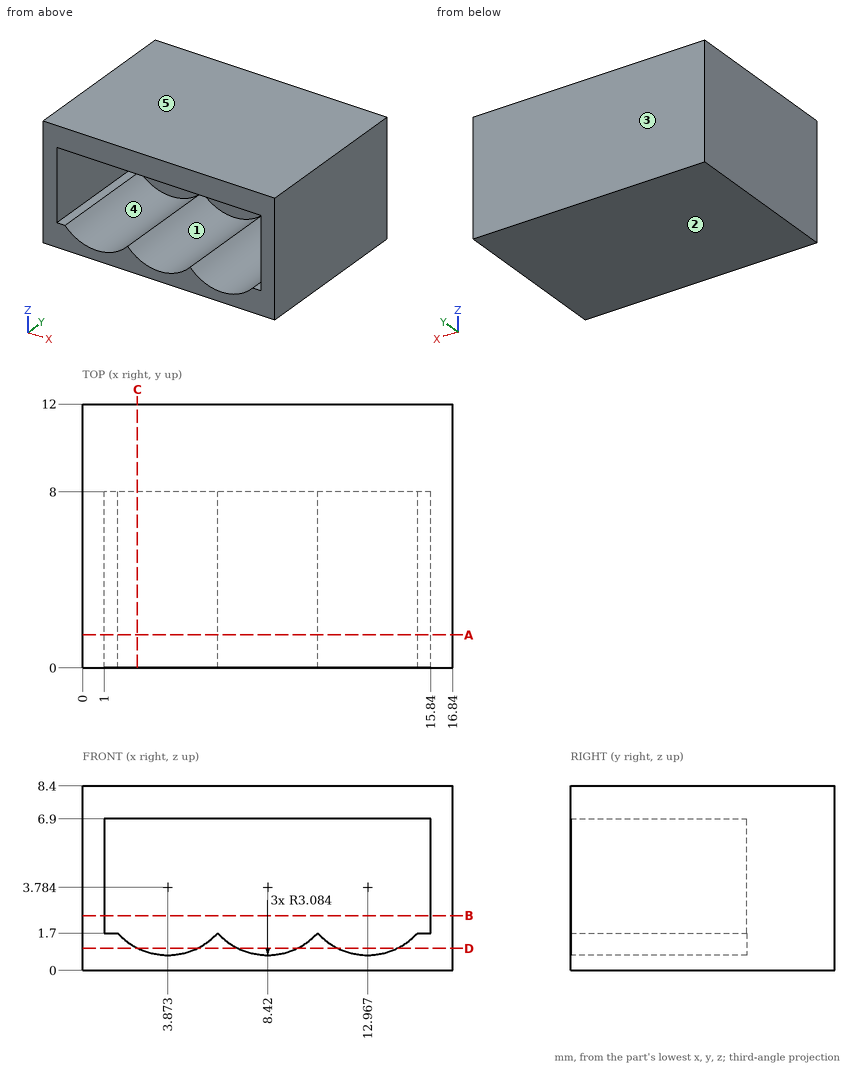
Job drawing, mm, ordinate dimensions from the low corner. One solid piece. A direction names the side the tool comes from. Give positions to 0.01 mm unless a question says otherwise; leave off trailing zeros. Write each loop counter-clockwise with the first axis right and the second up, starting at its lowest first coordinate (ties: lowest second). Pieces come first, ordered by that corner, then holes. Notation, with made-up numbers: M -35.75,-5.75 L -4.75,-5.75 A5 ccw -4.75,0.25 Z; hole C 58,-32 d5. An arc over 180 degrees is marked long. One line per item, written item: value. Start each with the question number.
Q1. Two-plate mould, pull along Z, no slides. Class the marked faces 3, 4 and 5: +Z half, -Z half, draft (parallel to the pull), parting line (faces both ways), or undercut.
Q2. Drop flat-ended pins along their axis: pin 1 Ø4 at (y, z) = (6, 4.5) entering from -X; pin 2 Ø1.9 at (x, z) = (6, 5) entering from -Y. Give the stop position or say it passes through.
Q3. Saw through at A-A, the plane y = 1.5. Write the cut outline in (x, z).
Q4. Saw through at B-B, the plane z = 2.5. Write the cut outline in (x, y).
Q5. Saw through at C-C, the plane x = 2.5. Write the cut outline in (y, z).
Q6. 3-axis set-ups, long thin cutter, end or side, ignore diameter. For the marked faces 1 and 2: which of +Z, -Z, +X, -X, +Y, -Y reach the whole face in a straight line?
Q7. Saw through at D-D, the plane z = 1. Write the cut outline in (x, y).
Q8. Probe probe 1 along X at (y, z) = (4.75, 5); probe 2 along Y at (x, z) = (9, 3.75); probe 3 along Z at (x, y) = (15, 7.25) (1 decimal). List the from-to ranges inside material, lowest first. Write a range as [from, to].
Output values:
1. face 3: draft
1. face 4: undercut
1. face 5: +Z half
2. pin 1: stops at x = 0
2. pin 2: stops at y = 8
3. outline: M 0,0 L 16.84,0 L 16.84,8.4 L 0,8.4 Z; hole M 1,1.7 L 1.6,1.7 A3.08 ccw 6.15,1.7 A3.08 ccw 10.69,1.7 A3.08 ccw 15.24,1.7 L 15.84,1.7 L 15.84,6.9 L 1,6.9 Z
4. outline: M 0,0 L 1,0 L 1,8 L 15.84,8 L 15.84,0 L 16.84,0 L 16.84,12 L 0,12 Z
5. outline: M 0,0 L 12,0 L 12,8.4 L 0,8.4 L 0,6.9 L 8,6.9 L 8,1.02 L 0,1.02 Z
6. face 1: -Y
6. face 2: -Z, +X, -X, +Y, -Y
7. outline: M 0,0 L 2.55,0 L 2.55,8 L 5.2,8 L 5.2,0 L 7.09,0 L 7.09,8 L 9.75,8 L 9.75,0 L 11.64,0 L 11.64,8 L 14.29,8 L 14.29,0 L 16.84,0 L 16.84,12 L 0,12 Z
8. probe 1: x = [0, 1], [15.84, 16.84]
8. probe 2: y = [8, 12]
8. probe 3: z = [0, 1.5], [6.9, 8.4]
